```python
from build123d import *

# Parameters (mm, degrees)
SKETCH_1_R          = 4
EXTRUDE_1_DEPTH     = 6.5
SKETCH_2_R          = 2.4
CUT_EXTRUDE_1_DEPTH = 13


with BuildPart() as part:
    # 草图1 → 凸台-拉伸1 (new, symmetric)
    with BuildSketch(Plane.XY):
        with BuildLine():
            Line((-27.5, 0), (27.5, 0))
            Line((27.5, 0), (27.5, 5))
            Line((27.5, 5), (17.69099654, 5))
            Line((17.69099654, 5), (14.005924481, 18.752876154))
            ThreePointArc((14.005924481, 18.752876154), (0, 29.5), (-14.005924481, 18.752876154))
            Line((-14.005924481, 18.752876154), (-17.69099654, 5))
            Line((-17.69099654, 5), (-27.5, 5))
            Line((-27.5, 5), (-27.5, 0))
        make_face()
        with Locations(Location((0, 15, 0), (0, 0, 180))):
            Circle(SKETCH_1_R, mode=Mode.SUBTRACT)
    extrude(amount=EXTRUDE_1_DEPTH, both=True)

    # 草图2 → 切除-拉伸1 (cut)
    with BuildSketch(Plane(origin=(0, 5, 0), x_dir=(1, 0, 0), z_dir=(0, 1, 0))):
        with Locations(Location((-21, 0, 0), (0, 0, 180))):
            Circle(SKETCH_2_R)
        with Locations(Location((21, 0, 0), (0, 0, 180))):
            Circle(SKETCH_2_R)
    extrude(amount=-CUT_EXTRUDE_1_DEPTH, mode=Mode.SUBTRACT)


solid = part.part
```
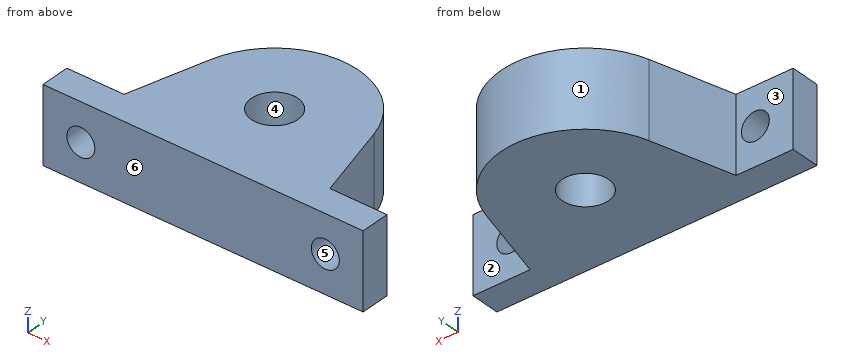
Check sheet for the modelled part. Datum: model origin and axes. Units: mm. Face numbers are marked on the shaded views. A direction names the side the tool comes from. Coordinates: 2 decimals unless noted, no trailing zeros. Order: outer loops, then holes, each group sorted by start corner. A loop starts at its lowest first (then second) coordinate and runs counter-clockwise, first axis right, second up. Notation, with made-up numbers: M -33,14.5 L -20,14.5 A29 cw -20,44.5 Z; hole C -6.5,7.5 d1. An arc over 180 degrees is marked long. Write each question's results on one line, items separated by ' | '. Start each with the question number.
1. Mould release check, pull along Y, two halves, no side actions. Record for the marked faces 4, 5 and 6: +Y half, -Y half, draft (parallel to the pull), parting line (faces both ways), or undercut.
2. Cross-section at D-D on y = 3.5. Record the cut outline in (x, z), and give its area (3 significant figures).
3. Cross-section at B-B on x = 0. Record the cut outline in (y, z).
4. Access from +Z, -Z, +X, -X, +Y, -Y to the whole of each face (thin tool, end or side, straight path). Record for the marked faces 1, 2 and 3.
5. Cross-section at A-A on z = 0. Record the cut outline in (x, y), and give its area (3 significant figures).
6. Material ranges on probe 1 along Z at (x, y) = (21, 3.5); probe 2 along Y at (x, z) = (24.5, -5); probe 3 along X at (y, z) = (16.5, 4), recorded low to high.
7. Cross-section at C-C on z = 3.5. Record the cut outline in (x, y).
8. Go/stop test with flat-tipped pins: P1, Ø1, axis at y = 18, z = -2, coming from the +X side; P2, Ø5, axis at x = -21, z = -2, coming from the +Y side; P3, Ø6, axis at y = 17.5, z = -3, coming from the -X side. Record where each tip stops, or that it passes through.
Checks:
1) face 4: undercut | face 5: draft | face 6: -Y half
2) outline: M -27.5,-6.5 L 27.5,-6.5 L 27.5,6.5 L -27.5,6.5 Z; hole C -21,0 d4.8; hole C 21,0 d4.8 | area: 679 mm²
3) outline: M 0,-6.5 L 11,-6.5 L 11,6.5 L 0,6.5 Z; M 19,-6.5 L 29.5,-6.5 L 29.5,6.5 L 19,6.5 Z
4) face 1: +Z, -Z, +Y | face 2: +Z, -Z, +X, +Y | face 3: +Z, -Z, -X, +Y
5) outline: M -27.5,0 L -23.4,0 L -23.4,5 L -27.5,5 Z; M -18.6,0 L 18.6,0 L 18.6,5 L 17.69,5 L 14.01,18.75 A14.5 ccw -14.01,18.75 L -17.69,5 L -18.6,5 Z; M 23.4,0 L 27.5,0 L 27.5,5 L 23.4,5 Z; hole C 0,15 d8 | area: 835 mm²
6) probe 1: z = -6.5 to -2.4, 2.4 to 6.5 | probe 2: y = 0 to 5 | probe 3: x = -14.61 to -3.71, 3.71 to 14.61
7) outline: M -27.5,0 L 27.5,0 L 27.5,5 L 17.69,5 L 14.01,18.75 A14.5 ccw -14.01,18.75 L -17.69,5 L -27.5,5 Z; hole C 0,15 d8
8) P1: stops at x = 14.34 | P2: stops at y = 5 | P3: stops at x = -15.15
